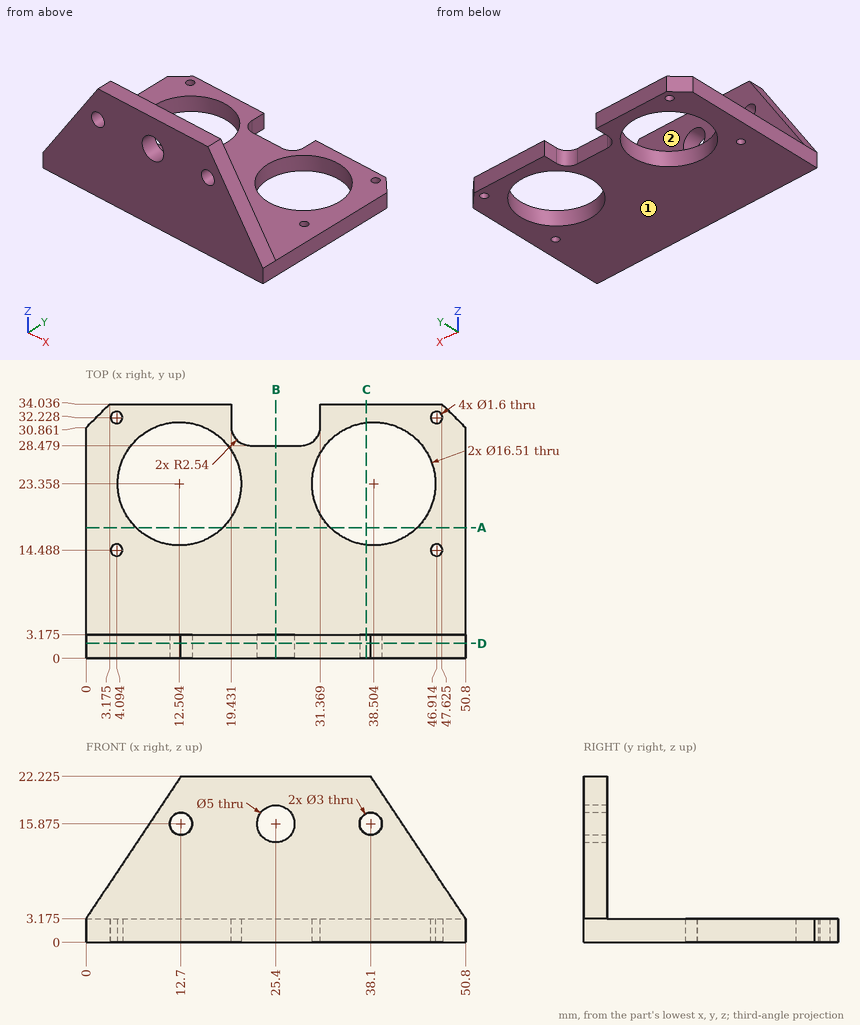
Part print with two shaded views. Sizes in mm from the minimum x, y, z corner. A direction names the side the tool comes from. Round coordinates to 2 decimals unless told otherwise and drop trailing zeros. Loops run counter-clockwise (first coordinate to the right, second up) from the corner with the lowest first, then second, coordinate; pieces in that order, holes last.
1. Slice it at D-D (y = 2). Give the cut face in (x, z) (3 decimals).
Solutions:
outline: (0, 0) - (50.8, 0) - (50.8, 3.175) - (38.1, 22.225) - (12.7, 22.225) - (0, 3.175) - close; hole circle Ø3 at (12.7, 15.875); hole circle Ø5 at (25.4, 15.875); hole circle Ø3 at (38.1, 15.875)
2. Flat gauge pins, fed straight in: pin 1 (1 mm diameter, centred on x = 46.914, y = 32.228, fed in from -Z); pin 2 (3.5 mm diameter, centred on x = 24.5, z = 2, fed in from +Y); pin 3 (4 mm diameter, centred on x = 33.5, z = 11.5, fed in from +Y) (3 decimals); pin 4 (1.5 mm diameter, centred on y = 33, z = 1.5, fed in from +X). Where does each tip first touch, or does it go through?
Solutions:
pin 1: passes through
pin 2: stops at y = 28.48
pin 3: stops at y = 3.175
pin 4: stops at x = 49.41
3. Drill centre lines: line 1 along Y through (x, z) = (22, 19.75) (3 decimals); line 2 along X through (y, z) = (3, 9.5). Where is each one in solid material? Low to high.
Solutions:
line 1: y = 0 to 3.175
line 2: x = 4.22 to 46.58
4. Slice it at A-A (y = 17.5). Give the cut face in (x, z) (3 decimals).
Solutions:
outline: (0, 0) - (6.688, 0) - (6.688, 3.175) - (0, 3.175) - close; (18.32, 0) - (32.688, 0) - (32.688, 3.175) - (18.32, 3.175) - close; (44.32, 0) - (50.8, 0) - (50.8, 3.175) - (44.32, 3.175) - close
5. Slice it at C-C (x = 37.5). Give the cut face in (y, z) (1 decimal), and give its area (3 significant figures).
Solutions:
outline: (0, 0) - (15.2, 0) - (15.2, 3.2) - (3.2, 3.2) - (3.2, 14.5) - (0, 14.5) - close; (0, 17.2) - (3.2, 17.2) - (3.2, 22.2) - (0, 22.2) - close; (31.6, 0) - (34, 0) - (34, 3.2) - (31.6, 3.2) - close
area: 108 mm2
6. Slice it at B-B (x = 25.4). Give the cut face in (y, z) (3 decimals), and give its area (3 significant figures).
Solutions:
outline: (0, 0) - (28.479, 0) - (28.479, 3.175) - (3.175, 3.175) - (3.175, 13.375) - (0, 13.375) - close; (0, 18.375) - (3.175, 18.375) - (3.175, 22.225) - (0, 22.225) - close
area: 135 mm2
7. 3-axis set-ups, long thin cutter, end or side, ignore diameter. For the marked faces 1 and 2: which of +Z, -Z, +X, -X, +Y, -Y reach the whole face in a straight line?
Solutions:
face 1: -Z, +X, -X, +Y, -Y
face 2: +Z, +X, -X, +Y
